Autodesk Inventor part; units mm, degrees
ref_plane "YZ Plane" through (0, 0, 0) normal (1, 0, 0) x (0, 1, 0)
ref_plane "XZ Plane" through (0, 0, 0) normal (0, 1, 0) x (-1, 0, 0)
ref_plane "XY Plane" through (0, 0, 0) normal (0, 0, 1) x (1, 0, 0)
sketch "Sketch1" plane through (0, 0, 0) normal (0, 0, 1) x (1, 0, 0)
  line L0 (0, 0) -> (4.7625, 0)
  line L1 (4.7625, 3.1115) -> (3.9687, 3.1115) construction
  line L2 (0, 3.1115) -> (0, 0)
  line L3 (4.7625, 0) -> (12.7, 0)
  line L4 (12.7, 0) -> (12.7, 3.1115) construction
  line L5 (12.7, 5.1753) -> (11.1125, 5.1753) construction
  line L6 (4.7625, 5.1753) -> (4.7625, 3.1115) construction
  line L7 (2.3812, 3.1115) -> (2.3812, 0) construction
  line L8 (8.7312, 5.1753) -> (8.7312, 0) construction
  line L9 (2.3812, 3.1115) -> (2.3812, 5.4927) construction
  circle A0 centre (2.3812, 5.4927) radius 2.3812 construction
  line L10 (6.35, 5.1753) -> (6.35, 0) construction
  line L11 (11.1125, 5.1753) -> (11.1125, 0) construction
  line L12 (4.7625, 3.1115) -> (12.7, 3.1115) construction
  line L13 (6.35, 5.1753) -> (4.7625, 5.1753) construction
  line L14 (4.7625, 3.1115) -> (4.7625, 0) construction
  line L15 (11.1125, 5.1753) -> (10.3187, 5.1753) construction
  line L16 (12.7, 3.1115) -> (12.7, 5.1753) construction
  line L17 (8.7312, 5.1753) -> (8.7312, 7.5565) construction
  circle A1 centre (8.7312, 7.5565) radius 2.3813 construction
  line L18 (0.7937, 3.1115) -> (0.7937, 0)
  line L19 (3.9687, 3.1115) -> (3.9687, 0)
  line L20 (7.1437, 5.1753) -> (7.1437, 0)
  line L21 (10.3187, 5.1753) -> (10.3187, 0)
  line L22 (3.9687, 3.1115) -> (0.7937, 3.1115)
  line L23 (0.7937, 3.1115) -> (0, 3.1115)
  line L24 (10.3187, 5.1753) -> (8.7312, 5.1753)
  line L25 (7.1437, 5.1753) -> (6.35, 5.1753) construction
  line L26 (8.7312, 5.1753) -> (7.1437, 5.1753)
  line L27 (3.9687, 3.1115) -> (7.1437, 5.1753)
  line L28 (0, 0) -> (0, 5.5563) construction
  line L29 (0, 5.5563) -> (17.4625, 5.5563) construction
  line L30 (0, 5.5563) -> (0, 7.9375) construction
  line L31 (0, 7.9375) -> (17.4625, 7.9375) construction
  line L32 (12.7, 3.1115) -> (13.4937, 3.1115) construction
  line L33 (12.7, 0) -> (17.4625, 0)
  line L34 (17.4625, 0) -> (17.4625, 3.1115)
  line L35 (15.0812, 0) -> (15.0812, 3.1115) construction
  line L36 (13.4937, 3.1115) -> (13.4937, 0)
  line L37 (16.6687, 3.1115) -> (16.6687, 0)
  line L38 (13.4937, 3.1115) -> (15.0812, 3.1115)
  line L39 (16.6687, 3.1115) -> (17.4625, 3.1115)
  line L40 (15.0812, 3.1115) -> (16.6687, 3.1115)
  line L41 (15.0812, 3.1115) -> (15.0812, 5.4928) construction
  line L42 (10.3187, 5.1753) -> (13.4937, 3.1115)
  line L43 (0, -12.7) -> (0, 0) construction
  line L44 (0, -7.1437) -> (26.1938, -7.1437) construction
  line L45 (0, -4.7625) -> (26.1938, -4.7625) construction
  line L46 (26.1938, -4.7625) -> (26.1938, -7.1437) construction
  line L47 (26.1938, -7.1437) -> (26.1938, -12.7) construction
  line L48 (26.1938, -12.7) -> (0, -12.7) construction
  line L49 (26.1938, -6.35) -> (34.3852, -6.35) construction
  line L50 (26.1938, -12.7) -> (34.3852, -12.7) construction
  line L51 (34.3852, -12.7) -> (34.3852, -6.35) construction
  line L52 (16.6688, -4.7625) -> (16.6688, -12.7) construction
  circle A2 centre (16.6688, -5.1435) radius 2.3813 construction
  circle A3 centre (16.6688, -7.2073) radius 2.3813 construction
  circle A4 centre (10.3187, -5.1435) radius 2.3813 construction
  circle A5 centre (10.3187, -7.2073) radius 2.3813 construction
  line L53 (10.3187, -4.7625) -> (10.3187, -12.7) construction
  line L54 (0, -7.5248) -> (26.1938, -7.5248) construction
  line L55 (8.7312, -7.5248) -> (8.7312, -12.7) construction
  line L56 (5.5562, -7.5248) -> (5.5562, -12.7) construction
  line L57 (18.2563, -7.5248) -> (18.2563, -12.7) construction
  line L58 (21.4313, -7.5248) -> (21.4313, -12.7) construction
  line L59 (0, -9.5885) -> (26.1938, -9.5885) construction
  line L60 (5.5562, -9.5885) -> (8.7312, -7.5248) construction
  line L61 (18.2563, -7.5248) -> (21.4312, -9.5885) construction
  line L62 (11.9062, -7.5248) -> (11.9062, -12.7) construction
  line L63 (15.0812, -7.5248) -> (15.0812, -12.7) construction
  line L64 (11.9062, -7.5248) -> (15.0812, -9.5885) construction
  line L65 (21.4313, -9.3266) -> (34.3852, -9.3266) construction
  line L66 (24.6063, -9.3266) -> (24.6063, -12.7) construction
  line L67 (21.4313, -9.3266) -> (20.1197, -7.1437) construction
  line L68 (26.1938, -9.5885) -> (30.9563, -9.5885) construction
  line L69 (30.9563, -9.5885) -> (30.9563, -12.7) construction
  line L70 (31.75, -9.3266) -> (31.75, -12.7) construction
  line L71 (31.75, -12.7) -> (29.723, -9.3266) construction
  line L72 (0, -4.7625) -> (-1.5875, -4.7625) construction
  line L73 (-1.5875, -4.7625) -> (-1.5875, -9.3266) construction
  line L74 (-1.5875, -9.3266) -> (5.5562, -9.3266) construction
  line L75 (1.4233, 7.874) -> (3.7622, 7.874)
  line L76 (5.5562, 3.1115) -> (7.1437, 5.1753)
  line L77 (10.3187, 5.1753) -> (11.9062, 3.1115)
  line L78 (11.9062, 3.1115) -> (13.4937, 3.1115)
  line L79 (5.5562, 3.1115) -> (3.9687, 3.1115)
  dimension "d8" = 6.35
  dimension "d9" = 5.1753
  dimension "d10" = 4.7625
  dimension "d11" = 2.3813
  dimension "d12" = 3.175
  dimension "d13" = 3.175
  dimension "d14" = 4.7625
  dimension "d15" = 2.3813
  dimension "d16" = 3.1115
  dimension "d17" = 5.5563
  dimension "d18" = 7.9375
  dimension "d19" = 6.35
  dimension "d20" = 3.175
  dimension "d21" = 2.3813
  dimension "d25" = 12.7
  dimension "d26" = 5.5563
  dimension "d27" = 7.9375
  dimension "d28" = 26.1938
  dimension "d29" = 8.1915
  dimension "d30" = 6.35
  dimension "d33" = 9.525
  dimension "d35" = 0.381
  dimension "d36" = 0.0635
  dimension "d38" = 6.35
  dimension "d39" = 0.381
  dimension "d40" = 0.381
  dimension "d41" = 0.0635
  dimension "d42" = 0.0635
  dimension "d43" = 9.525
  dimension "d46" = 1.5875
  dimension "d47" = 4.7625
  dimension "d48" = 1.5875
  dimension "d49" = 4.7625
  dimension "d50" = 3.1115
  dimension "d51" = 1.5875
  dimension "d52" = 4.7625
  dimension "d53" = 3.3734
  dimension "d54" = 3.175
  dimension "d55" = 31
  dimension "d56" = 9.525
  dimension "d57" = 9.525
  dimension "d59" = 0.7937
  dimension "d60" = 31
  dimension "d61" = 1.5875
  dimension "d62" = 3.3734
  dimension "d63" = 0.0635
  dimension "d70" = 0.7937
  dimension "d71" = 0.7937
extrude "Extrusion1" add sketch "Sketch1" along normal blind 25.4 contours L2 L23 L18 L0 | L18 L22 L19 L0 | L19 L79 L76 L20 L3 L0 | L20 L26 L24 L21 L3 | L21 L77 L78 L36 L33 L3 | L36 L38 L40 L37 L33
sketch "Sketch2" plane through (16.6687, 0, 0) normal (1, 0, 0) x (0, 0, -1)
  line L0 (0, 0) -> (0, 3.1115)
  line L1 (0, 3.1115) -> (-25.4, 3.1115)
  line L2 (-25.4, 0) -> (-25.4, 3.1115)
  line L3 (0, 0) -> (-25.4, 0)
extrude "Extrusion2" add sketch "Sketch2" along normal blind 25.4
sketch "Sketch3" plane through (0, 0, 0) normal (-1, 0, 0) x (0, 0, 1)
  line L0 (0, 3.1115) -> (0, 0)
  line L1 (0, 0) -> (25.4, 0)
  line L2 (25.4, 3.1115) -> (25.4, 0)
  line L3 (0, 3.1115) -> (25.4, 3.1115)
extrude "Extrusion3" add sketch "Sketch3" along normal blind 25.4
fillet "Fillet1" radius 2.54 4 edges at (10.3187, 5.1753, 12.7) (7.1437, 5.1753, 12.7) (11.9062, 3.1115, 12.7) (5.5562, 3.1115, 12.7)
equation "\"d19\" = d8"
equation "\"d26\" = d17"
equation "\"d27\" = d18"
equation "\"d39\" = d35"
equation "\"d40\" = d39"
equation "\"d41\" = d36"
equation "\"d42\" = d41"
equation "\"d50\" = d16"
equation "\"d51\" = d46"
equation "\"d52\" = d47"
equation "\"d57\" = d56"
equation "\"d60\" = d55"
equation "\"d62\" = d53"
properties part number "Sketch - Ball Shifting Shaft"
Part model, mm, in its own coordinate system. A direction names the side the tool comes from. Coordinates: 2 decimals unless noted, no trailing zeros. Order: outer loops, then holes, each group sorted by start corner. A loop starts at its lowest first (then second) coordinate and runs counter-clockwise, first axis right, second up. Notation, with made-up numbers: (-5, 70.5) -> (25, 70.5) arc R6 ccw to (25, 74.5) -> close; hole circle Ø11 at (5.5, -38). An arc over 180 degrees is marked (long way). Put each result on its own line as item: value. Start each with the question number.
(1) Pin check, flat tip, straight feed: pin 1 Ø8 at (x, z) = (-9.5, 21.5) entering from +Y. Stop position of the tip, or through.
(2) Band-saw the part on C-C (x = 10). Give the cut face in (y, z).
(3) Probe line 1 along Y through (x, z) = (0, 7); line 2 along X through (y, z) = (4.1, 10); line 3 along X through (y, z) = (4.55, 19.5). List the from-to ranges inside material, lowest first. Write a range as [from, to].
(4) Band-saw the part on B-B (x = 2.5). Give the cut face in (y, z), then the cut area to 3 significant figures.
(5) Band-saw the part on A-A (z = 13.5). Give the cut face in (x, y), then the cut area to 3 significant figures.
(6) Which spindle directions (+Z, -Z, +X, -X, +Y, -Y) get a long thin tool onto all of the face, cutting with end or side? Do faces 1 (the face through (-10, 3.112, 13)), 2 (the face through (9, 1, 0)), 3 (the face through (27, 3.112, 13)). Say none if no direction does.
Determined:
1. pin 1: stops at y = 3.11
2. outline: (0, 0) -> (5, 0) -> (5, 25.4) -> (0, 25.4) -> close
3. line 1: y = [0, 3.11]
3. line 2: x = [6.32, 11.15]
3. line 3: x = [6.73, 10.74]
4. outline: (0, 0) -> (3.11, 0) -> (3.11, 25.4) -> (0, 25.4) -> close
4. area: 79.0 mm²
5. outline: (-25.4, 0) -> (42.07, 0) -> (42.07, 3.11) -> (13.16, 3.11) arc R2.54 cw to (11.14, 4.1) -> (11.08, 4.18) arc R2.54 ccw to (9.07, 5.18) -> (8.39, 5.18) arc R2.54 ccw to (6.38, 4.18) -> (6.32, 4.1) arc R2.54 cw to (4.31, 3.11) -> (-25.4, 3.11) -> close
5. area: 220 mm²
6. face 1: +Z, -Z, -X, +Y
6. face 2: -Z, +X, -X, +Y, -Y
6. face 3: +Z, -Z, +X, +Y
